Build history of the part. All positions in model axes, mm. Face numbers are marked on the shaded views. Round coordinates to 2 decimals unless told otherwise and drop trailing zeros. Write each loop counter-clockwise with the first axis right and the second up, starting at its lowest first coordinate (ties: lowest second). Pieces come first, ordered by that corner, then holes.
Item 1: Band-saw the part on C-C, the plane z = 8. Write the cut outline in (x, y).
Item 2: Wall check: probe 1 along Y at (x, z) = (18.65, 2.5); probe 2 along Y at (x, z) = (0, 8). Give the ranges that are in metal, low to high.
Item 3: Mould opens along Y. For the marked faces 1, 2 and 3 say: +Y half, -Y half, draft (parallel to the pull), parting line (faces both ways), or undercut.
Item 4: Band-saw the part on D-D, the plane y = -18.65. Write the cut outline in (x, z).
Item 5: Band-saw the part on A-A, the plane y = 0. Write the cut outline in (x, z), then the cut area to 3 significant figures.
Item 6: Drop flat-ended pins along their axis: pin 1 Ø4.5 at (x, y) = (18.65, -18.65) entering from -Z; pin 2 Ø3.5 at (x, y) = (-18.65, -18.65) entering from -Z. Give the stop position or say it passes through.
```python
from build123d import *

# Parameters (mm, degrees)
SKETCH1_W               = 50
SKETCH1_H               = 50
BOSS_EXTRUDE1_DEPTH     = 11.5
SKETCH2_R               = 1.984375
CUT_EXTRUDE1_DEPTH      = 12.5
MIRROR2_COPY_1_SKETCH_R = 1.984375
MIRROR2_COPY_1_DEPTH    = 12.5
SKETCH3_R               = 4.2164
CUT_EXTRUDE2_DEPTH      = 12.5


with BuildPart() as part:
    # Sketch1 → Boss-Extrude1 (new body)
    with BuildSketch(Plane.XY):
        Rectangle(SKETCH1_W, SKETCH1_H)
    extrude(amount=BOSS_EXTRUDE1_DEPTH)

    # Sketch2 → Cut-Extrude1 (cut, through all)
    with BuildSketch(Plane.XY.offset(11.5)):
        with Locations((-18.65, 18.65)):
            Circle(SKETCH2_R)
    cut_extrude1 = extrude(amount=-CUT_EXTRUDE1_DEPTH, mode=Mode.SUBTRACT)

    # Mirror1: Cut-Extrude1 across plane
    add(cut_extrude1.mirror(Plane.ZX), mode=Mode.SUBTRACT)

    # Mirror2: Cut-Extrude1 across plane
    add(cut_extrude1.mirror(Plane(origin=(0, 0, 0), x_dir=(0, 0, 1), z_dir=(1, 0, 0))), mode=Mode.SUBTRACT)

    # Mirror2 copy 1 sketch → Mirror2 copy 1 (cut, through all)
    with BuildSketch(Plane(origin=(0, 0, 11.5), x_dir=(-1, 0, 0), z_dir=(0, 0, 1))):
        with Locations((-18.65, 18.65)):
            Circle(MIRROR2_COPY_1_SKETCH_R)
    extrude(amount=-MIRROR2_COPY_1_DEPTH, mode=Mode.SUBTRACT)

    # Sketch3 → Cut-Extrude2 (cut, through all)
    with BuildSketch(Plane.XY.offset(11.5)):
        Circle(SKETCH3_R)
    extrude(amount=-CUT_EXTRUDE2_DEPTH, mode=Mode.SUBTRACT)


solid = part.part
```
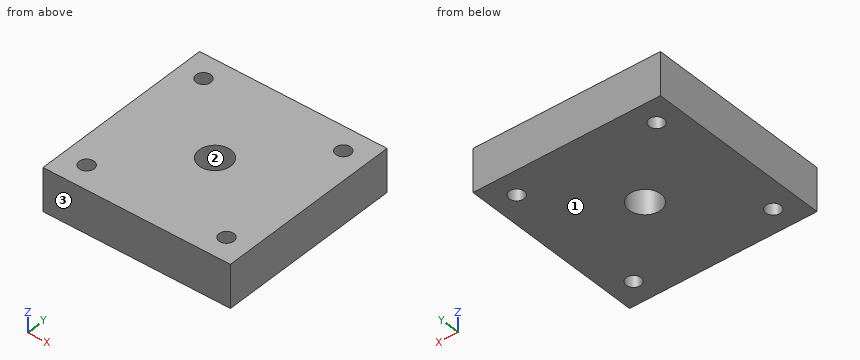
Results:
1. outline: (-25, -25) - (25, -25) - (25, 25) - (-25, 25) - close; hole circle Ø3.97 at (-18.65, -18.65); hole circle Ø3.97 at (-18.65, 18.65); hole circle Ø8.43 at (0, 0); hole circle Ø3.97 at (18.65, -18.65); hole circle Ø3.97 at (18.65, 18.65)
2. probe 1: y = -25 to -20.63, -16.67 to 16.67, 20.63 to 25
2. probe 2: y = -25 to -4.22, 4.22 to 25
3. face 1: draft
3. face 2: undercut
3. face 3: -Y half
4. outline: (-25, 0) - (-20.63, 0) - (-20.63, 11.5) - (-25, 11.5) - close; (-16.67, 0) - (16.67, 0) - (16.67, 11.5) - (-16.67, 11.5) - close; (20.63, 0) - (25, 0) - (25, 11.5) - (20.63, 11.5) - close
5. outline: (-25, 0) - (-4.22, 0) - (-4.22, 11.5) - (-25, 11.5) - close; (4.22, 0) - (25, 0) - (25, 11.5) - (4.22, 11.5) - close
5. area: 478 mm2
6. pin 1: stops at z = 0
6. pin 2: passes through
